from build123d import *

# Parameters (mm, degrees)
SKETCH_2_R      = 4
SKETCH_2_R_2    = 1.25
SKETCH_2_R_3    = 1.5
EXTRUDE_1_DEPTH = 2
FILLET_1_R      = 0.1


with BuildPart() as part:
    # Эскиз2 → Бобышка-Вытянуть1 (new body)
    with BuildSketch(Plane.XY):
        with BuildLine():
            Line((-9.75, 16.5), (-9.75, 12.523623513))
            ThreePointArc((-9.75, 12.523623513), (0, 10.5), (9.75, 12.523623513))
            Line((9.75, 12.523623513), (9.75, 16.5))
            Line((9.75, 16.5), (11.75, 16.5))
            Line((11.75, 16.5), (11.75, 18.5))
            Line((11.75, 18.5), (9.75, 18.5))
            Line((9.75, 18.5), (9.75, 21.106870919))
            ThreePointArc((9.75, 21.106870919), (16.440232663, 16.440232663), (21.106870919, 9.75))
            Line((21.106870919, 9.75), (18.5, 9.75))
            Line((18.5, 9.75), (18.5, 11.75))
            Line((18.5, 11.75), (16.5, 11.75))
            Line((16.5, 11.75), (16.5, 9.75))
            Line((16.5, 9.75), (12.523623513, 9.75))
            ThreePointArc((12.523623513, 9.75), (10.5, 0), (12.523623513, -9.75))
            Line((12.523623513, -9.75), (16.5, -9.75))
            Line((16.5, -9.75), (16.5, -11.75))
            Line((16.5, -11.75), (18.5, -11.75))
            Line((18.5, -11.75), (18.5, -9.75))
            Line((18.5, -9.75), (21.106870919, -9.75))
            ThreePointArc((21.106870919, -9.75), (16.440232663, -16.440232663), (9.75, -21.106870919))
            Line((9.75, -21.106870919), (9.75, -18.5))
            Line((9.75, -18.5), (11.75, -18.5))
            Line((11.75, -18.5), (11.75, -16.5))
            Line((11.75, -16.5), (9.75, -16.5))
            Line((9.75, -16.5), (9.75, -12.523623513))
            ThreePointArc((9.75, -12.523623513), (0, -10.5), (-9.75, -12.523623513))
            Line((-9.75, -12.523623513), (-9.75, -16.5))
            Line((-9.75, -16.5), (-11.75, -16.5))
            Line((-11.75, -16.5), (-11.75, -18.5))
            Line((-11.75, -18.5), (-9.75, -18.5))
            Line((-9.75, -18.5), (-9.75, -21.106870919))
            ThreePointArc((-9.75, -21.106870919), (-16.440232663, -16.440232663), (-21.106870919, -9.75))
            Line((-21.106870919, -9.75), (-18.5, -9.75))
            Line((-18.5, -9.75), (-18.5, -11.75))
            Line((-18.5, -11.75), (-16.5, -11.75))
            Line((-16.5, -11.75), (-16.5, -9.75))
            Line((-16.5, -9.75), (-12.523623513, -9.75))
            ThreePointArc((-12.523623513, -9.75), (-10.5, 0), (-12.523623513, 9.75))
            Line((-12.523623513, 9.75), (-16.5, 9.75))
            Line((-16.5, 9.75), (-16.5, 11.75))
            Line((-16.5, 11.75), (-18.5, 11.75))
            Line((-18.5, 11.75), (-18.5, 9.75))
            Line((-18.5, 9.75), (-21.106870919, 9.75))
            ThreePointArc((-21.106870919, 9.75), (-16.440232663, 16.440232663), (-9.75, 21.106870919))
            Line((-9.75, 21.106870919), (-9.75, 18.5))
            Line((-9.75, 18.5), (-11.75, 18.5))
            Line((-11.75, 18.5), (-11.75, 16.5))
            Line((-11.75, 16.5), (-9.75, 16.5))
        make_face()
        Circle(SKETCH_2_R, mode=Mode.SUBTRACT)
        with Locations((0, 7.5)):
            Circle(SKETCH_2_R_2, mode=Mode.SUBTRACT)
        with Locations((5.303300859, 5.303300859)):
            Circle(SKETCH_2_R_2, mode=Mode.SUBTRACT)
        with Locations((7.5, 0)):
            Circle(SKETCH_2_R_2, mode=Mode.SUBTRACT)
        with Locations((5.303300859, -5.303300859)):
            Circle(SKETCH_2_R_2, mode=Mode.SUBTRACT)
        with Locations((0, -7.5)):
            Circle(SKETCH_2_R_2, mode=Mode.SUBTRACT)
        with Locations((-5.303300859, -5.303300859)):
            Circle(SKETCH_2_R_2, mode=Mode.SUBTRACT)
        with Locations((-7.5, 0)):
            Circle(SKETCH_2_R_2, mode=Mode.SUBTRACT)
        with Locations((-5.303300859, 5.303300859)):
            Circle(SKETCH_2_R_2, mode=Mode.SUBTRACT)
        with Locations((13.825687912, 13.825687912)):
            Circle(SKETCH_2_R_3, mode=Mode.SUBTRACT)
        with Locations((13.825687912, -13.825687912)):
            Circle(SKETCH_2_R_3, mode=Mode.SUBTRACT)
        with Locations((-13.825687912, -13.825687912)):
            Circle(SKETCH_2_R_3, mode=Mode.SUBTRACT)
        with Locations((-13.825687912, 13.825687912)):
            Circle(SKETCH_2_R_3, mode=Mode.SUBTRACT)
    extrude(amount=EXTRUDE_1_DEPTH)

    # Скругление1
    fillet_1_edges = [part.edges().sort_by_distance(p)[0] for p in [
        (16.440232663, -16.440232663, 2),
        (16.440232663, 16.440232663, 2),
        (16.440232663, -16.440232663, 0),
        (-16.440232663, -16.440232663, 0),
        (-16.440232663, 16.440232663, 0),
        (16.440232663, 16.440232663, 0),
        (-16.440232663, 16.440232663, 2),
        (-16.440232663, -16.440232663, 2),
    ]]
    fillet(fillet_1_edges, radius=FILLET_1_R)


solid = part.part
The listing builds one solid part. Answer for the finished solid, in the listing's coordinates (mm). A direction names the side the tool comes from. Give positions to 0.01 mm unless a question says otherwise; leave off trailing zeros. Loops run counter-clockwise (first coordinate to the right, second up) from the corner with the lowest first, then second, coordinate; pieces in that order, holes last.
Item 1: A cutting plane is placed at D-D (z = 0.8). Give the number of separate pieces and of enclosed holes in the cut face, then the cut area to 3 significant figures.
Derived:
separate pieces: 1
enclosed holes: 13
area: 660 mm2
Item 2: A cutting plane is placed at B-B (x = 7.5). Give the vertices of the cut face in (y, z).
Derived:
outline: (-11.68, 0) - (-1.25, 0) - (-1.25, 2) - (-11.68, 2) - close; (1.25, 0) - (11.68, 0) - (11.68, 2) - (1.25, 2) - close
Item 3: A tool of negligible diameter and unlimited length cuts with its end or side. For faces 1 (the cylindrical face through (-16.36, -16.52, 0.99)), 2 (the flat face through (-9.75, 15, 1)), 3 (the flat face through (-15, -9.75, 1)), 4 (the flat face through (-11, 16.5, 1)), from which of +Z, -Z, +X, -X, +Y, -Y can it reach the whole face along a straight path? Write none if from no direction.
Derived:
face 1: +Z, -Z, -X, -Y
face 2: +Z, -Z, +Y
face 3: +Z, -Z, -X
face 4: +Z, -Z
Item 4: Each of these flat-tipped pins is pushed along its axis until it touches: pin 1 Ø2 at (x, y) = (-5.3, 5.3) entering from +Z; pin 2 Ø1 at (y, z) = (-14, 1.5) entering from +X; pin 3 Ø0.6 at (y, z) = (-20.5, 1.5) entering from +X; pin 4 Ø1 at (x, z) = (17, 1) entering from -Y. Where does it stop, or does it pass through?
Derived:
pin 1: passes through
pin 2: stops at x = 18.93
pin 3: stops at x = 11.51
pin 4: stops at y = -16.38
Item 5: Find the intervals of material crossed by line 1 along X through (y, z) = (-10, 1.6); line 2 along Y through (x, z) = (-4.5, 1.2); line 3 along Y through (x, z) = (13, 1.2), in increasing order.
Derived:
line 1: x = -20.99 to -18.5, -16.5 to 16.5, 18.5 to 20.99
line 2: y = -10.92 to -6.26, -4.35 to 4.35, 6.26 to 10.92
line 3: y = -19.28 to -15.08, -12.57 to -9.75, 9.75 to 12.57, 15.08 to 19.28
Item 6: A cutting plane is placed at A-A (y = 0). Give the vertices of the cut face in (x, z), then the cut area to 3 significant figures.
Derived:
outline: (-10.5, 0) - (-8.75, 0) - (-8.75, 2) - (-10.5, 2) - close; (-6.25, 0) - (-4, 0) - (-4, 2) - (-6.25, 2) - close; (4, 0) - (6.25, 0) - (6.25, 2) - (4, 2) - close; (8.75, 0) - (10.5, 0) - (10.5, 2) - (8.75, 2) - close
area: 16.0 mm2
Item 7: Determine the mould class of faces 5 (the cylindrical face through (6.25, 0.05, 0.99)), 6 (the flat face through (-9.75, -20, 1)), 7 (the cylindrical face through (0.1, -10.5, 1)), 8 (the cylindrical face through (-10.5, -0.1, 1)) for opening direction Y: +Y half, -Y half, draft (parallel to the pull), parting line (faces both ways), or undercut.
Derived:
face 5: undercut
face 6: draft
face 7: -Y half
face 8: undercut
